Part model, mm, in its own coordinate system. Face numbers are marked on the shaded views. A direction names the side the tool comes from. Coordinates: 2 decimals unless noted, no trailing zeros. Write each loop counter-clockwise with the first axis right and the second up, starting at its lowest first coordinate (ties: lowest second). Pieces come first, ordered by that corner, then holes. Notation, with made-up numbers: (11.25, 16) -> (18.25, 16) arc R37 ccw to (18.25, 55) -> close; hole circle Ø1 at (86, 76). An arc over 180 degrees is marked (long way). Write item = value, one per line.
from build123d import *

# Parameters (mm, degrees)
SKETCH3_R           = 4.5
BOSS_EXTRUDE1_DEPTH = 18
FILLET1_R           = 5
FILLET2_R           = 5
CUT_EXTRUDE2_DEPTH  = 19.0000001
SKETCH6_R           = 2
CUT_EXTRUDE3_DEPTH  = 19.0000001


with BuildPart() as part:
    # Sketch3 → Boss-Extrude1 (new body)
    with BuildSketch(Plane.XY):
        with BuildLine():
            Line((-31.929873349, -122.5), (31.929873349, -122.5))
            ThreePointArc((31.929873349, -122.5), (38.210043039, -120.281996444), (41.704324989, -114.611893732))
            Line((41.704324989, -114.611893732), (73.308387301, 31.660797012))
            ThreePointArc((73.308387301, 31.660797012), (0, 122.5), (-73.308387301, 31.660797012))
            Line((-73.308387301, 31.660797012), (-41.704324989, -114.611893732))
            ThreePointArc((-41.704324989, -114.611893732), (-38.210043039, -120.281996444), (-31.929873349, -122.5))
        make_face()
        with Locations((50, -12.5)):
            Circle(SKETCH3_R, mode=Mode.SUBTRACT)
        with Locations((50, 87.5)):
            Circle(SKETCH3_R, mode=Mode.SUBTRACT)
        with Locations((-50, 87.5)):
            Circle(SKETCH3_R, mode=Mode.SUBTRACT)
        with Locations((-50, -12.5)):
            Circle(SKETCH3_R, mode=Mode.SUBTRACT)
        with BuildLine():
            Line((-31.929873349, -112.5), (-51.284518999, -22.921132901))
            ThreePointArc((-51.284518999, -22.921132901), (-39.736825778, -10.282511582), (-55.472323677, -3.538768301))
            Line((-55.472323677, -3.538768301), (-63.533935661, 33.772690744))
            ThreePointArc((-63.533935661, 33.772690744), (-64.271528905, 57.204152316), (-56.648842383, 79.373322021))
            ThreePointArc((-56.648842383, 79.373322021), (-41.800877501, 80.940702001), (-43.531035666, 95.770580418))
            ThreePointArc((-43.531035666, 95.770580418), (0, 112.5), (43.531035666, 95.770580418))
            ThreePointArc((43.531035666, 95.770580418), (41.800877501, 80.940702001), (56.648842383, 79.373322021))
            ThreePointArc((56.648842383, 79.373322021), (64.271528905, 57.204152316), (63.533935661, 33.772690744))
            Line((63.533935661, 33.772690744), (55.472323677, -3.538768301))
            ThreePointArc((55.472323677, -3.538768301), (39.736825778, -10.282511582), (51.284518999, -22.921132901))
            Line((51.284518999, -22.921132901), (31.929873349, -112.5))
            Line((31.929873349, -112.5), (-31.929873349, -112.5))
        make_face(mode=Mode.SUBTRACT)
    extrude(amount=BOSS_EXTRUDE1_DEPTH)

    # Fillet1
    fillet1_edges = [part.edges().sort_by_distance(p)[0] for p in [
        (-31.929873349, -112.5, 9),
        (31.929873349, -112.5, 9),
    ]]
    fillet(fillet1_edges, radius=FILLET1_R)

    # Fillet2
    fillet2_edges = [part.edges().sort_by_distance(p)[0] for p in [
        (51.284518999, -22.921132901, 9),
        (55.472323677, -3.538768301, 9),
        (56.648842383, 79.373322021, 9),
        (43.531035666, 95.770580418, 9),
        (-43.531035666, 95.770580418, 9),
        (-56.648842383, 79.373322021, 9),
        (-55.472323677, -3.538768301, 9),
        (-51.284518999, -22.921132901, 9),
    ]]
    fillet(fillet2_edges, radius=FILLET2_R)

    # Sketch5 → Cut-Extrude2 (cut, through all)
    with BuildSketch(Plane.XY.offset(18)):
        Polygon((47.724403212, -39.39837277), (54.444339069, -31.972010438), (57.506356145, -41.47554836), (70.328868077, -126.043088926), (-63.485047771, -126.043088926), (-57.506356145, -41.47554836), (-54.443982463, -31.973660914), (-47.723687693, -39.401684395), align=None)
    extrude(amount=-CUT_EXTRUDE2_DEPTH, mode=Mode.SUBTRACT)

    # Sketch6 → Cut-Extrude3 (cut, through all)
    with BuildSketch(Plane.XY.offset(18)):
        with Locations((-70, 47.5)):
            Circle(SKETCH6_R)
        with Locations((70, 47.5)):
            Circle(SKETCH6_R)
    extrude(amount=-CUT_EXTRUDE3_DEPTH, mode=Mode.SUBTRACT)


solid = part.part
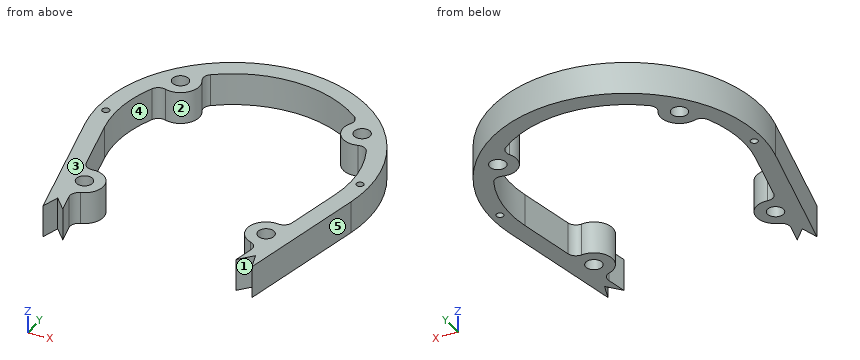
Q1. Pin check, flat tips, straight feed: pin 1 (4.5 mm diameter, centred on x = 70, y = 47.5, fed in from +Z); pin 2 (2 mm diameter, centred on x = 3.5, z = 11.5, fed in from -Y); pin 3 (3 mm diameter, centred on x = 13, z = 8.5, fed in from -Y); pin 4 (1.5 mm diameter, centred on x = -19, z = 10, fed in from +Y). Stop position of each tip, or through.
Model answer:
pin_1 = 18
pin_2 = 112.34
pin_3 = 110.86
pin_4 = 120.25
Q2. Saw through at A-A on x = -70. Give the cut face in (y, z).
Model answer:
outline = (16.35, 0) -> (45.5, 0) -> (45.5, 18) -> (16.35, 18) -> close; (49.5, 0) -> (74.43, 0) -> (74.43, 18) -> (49.5, 18) -> close
Q3. Which spindle directions (+Z, -Z, +X, -X, +Y, -Y) get a long thin tool onto all of the face, cutting with end or side? Do the marked faces 4 and 5. Say none if no direction does.
Model answer:
face_4 = +Z, -Z
face_5 = +Z, -Z, +X, -Y
Q4. Probe line 1 (X direction, y = 89, z = 4.75); line 2 (X direction, y = -16, z = 7); line 3 (X direction, y = 65, z = 3.5). List the from-to ranges inside material, lowest first. Write a range as from..to.
Model answer:
line_1 = -62.47..-54.24, -45.76..-39.61, 39.61..45.76, 54.24..62.47
line_2 = -63.01..-52.83, -47.17..-40.1, 40.1..47.17, 52.83..63.01
line_3 = -72.93..-62.6, 62.6..72.93
Q5. Saw through at B-B on y = 60.5. Give the cut face in (x, z).
Model answer:
outline = (-73.86, 0) -> (-63.69, 0) -> (-63.69, 18) -> (-73.86, 18) -> close; (63.69, 0) -> (73.86, 0) -> (73.86, 18) -> (63.69, 18) -> close
Q6. Saw through at D-D on z = 4. Count the separate pieces of the cut face and the enclosed holes in it, and give its area (3 significant figures).
Model answer:
separate_pieces = 1
enclosed_holes = 6
area = 4,530 mm²
Q7. Mould opens along Y. For the marked faces 1, 2 and 3 say: released by +Y, released by -Y, zero draft, split by the parting line, or undercut.
Model answer:
face_1 = released by -Y
face_2 = undercut
face_3 = zero draft
Q8. Saw through at C-C on y = -15. Give the cut face in (x, z), and give its area (3 significant figures).
Model answer:
outline = (-63.23, 0) -> (-53.74, 0) -> (-53.74, 18) -> (-63.23, 18) -> close; (-46.26, 0) -> (-39.8, 0) -> (-39.8, 18) -> (-46.26, 18) -> close; (39.8, 0) -> (46.26, 0) -> (46.26, 18) -> (39.8, 18) -> close; (53.74, 0) -> (63.23, 0) -> (63.23, 18) -> (53.74, 18) -> close
area = 574 mm²
